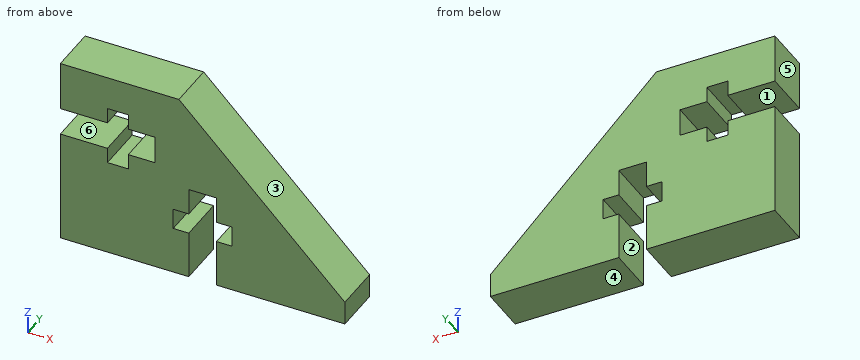
Autodesk Inventor part; units mm, degrees
ref_plane "Work Plane1" through (0, 0, 0) normal (0, 0, 1) x (1, 0, 0)
ref_plane "YZ Plane" through (0, 0, 0) normal (1, 0, 0) x (0, 1, 0)
ref_plane "XZ Plane" through (0, 0, 0) normal (0, 1, 0) x (-1, 0, 0)
ref_plane "Work Plane1" through (0, 0, 0) normal (0, 0, 1) x (1, 0, 0)
sketch "Sketch1" plane through (0, 0, 0) normal (0, 0, 1) x (1, 0, 0)
  line L0 (41.9864, 2.5) -> (43.4368, -2.0363) construction
  arc A0 (41.9864, 2.5) -> (43.4368, -2.0363) centre (41.9864, 0) ccw construction
  line L1 (112.0586, -28.575) -> (85.0037, -28.575) construction
  line L2 (112.0586, 28.1043) -> (112.0586, -28.575) construction
  line L3 (83.2959, 28.1043) -> (112.0586, 28.1043) construction
  arc A1 (83.2959, 28.1043) -> (1.0011, 28.575) centre (41.9864, 0) ccw construction
  line L4 (-116.5414, 28.575) -> (1.0011, 28.575) construction
  line L5 (-116.5414, -29.0493) -> (-116.5414, 28.575) construction
  line L6 (-0.7121, -29.0493) -> (-116.5414, -29.0493) construction
  arc A2 (-0.7121, -29.0493) -> (85.0037, -28.575) centre (41.9864, 0) ccw construction
  line L7 (-110.1914, 28.575) -> (-110.1914, 24.0792) construction
  line L8 (-111.9045, -9.9993) -> (-73.8045, -9.9993)
  line L9 (-73.8045, -9.9993) -> (-73.8045, -16.3493)
  line L10 (-73.8045, -16.3493) -> (-111.9045, -16.3493)
  line L11 (-111.9045, -16.3493) -> (-111.9045, -9.9993)
  circle A3 centre (88.3718, 12.2257) radius 1.8542
  circle A4 centre (108.8836, -22.6993) radius 1.8542
  circle A5 centre (-92.8545, -12.7) radius 1.8542
  circle A6 centre (-113.3664, 22.225) radius 1.8542
  circle A7 centre (-92.8545, 12.2257) radius 1.8542
  circle A8 centre (-113.3664, -22.6993) radius 1.8542
  circle A9 centre (88.3718, -12.7) radius 1.8542
  circle A10 centre (108.8836, 22.225) radius 1.8542
  point P0 (0, 0)
  dimension "d0" = 38.1
  dimension "d1" = 6.35
  dimension "d2" = 12.7
extrude "Extrusion1" add sketch "Sketch1" along normal blind 25.4 contours L8 L9 L10 L11 | A5
chamfer "Chamfer1" distance 22.225 angle 45 1 edges at (-73.8045, -13.1743, 25.4)
sketch "Sketch2" plane through (-111.9045, -16.3493, 0) normal (0, -1, 0) x (1, 0, 0)
  line L0 (38.1, 0) -> (0, 0)
  line L1 (17.1958, 0) -> (20.9042, 0)
  line L2 (19.05, 12.7239) -> (19.05, -0.6753) construction
  line L3 (17.1958, 12.7) -> (20.9042, 12.7)
  line L4 (20.9042, 12.7) -> (20.9042, 0)
  line L5 (20.9042, 0) -> (17.1958, 0)
  line L6 (17.1958, 0) -> (17.1958, 12.7)
  line L7 (15.113, 9.144) -> (22.987, 9.144)
  line L8 (22.987, 9.144) -> (22.987, 6.35)
  line L9 (22.987, 6.35) -> (15.113, 6.35)
  line L10 (15.113, 6.35) -> (15.113, 9.144)
  line L11 (0, 0) -> (0, 25.4)
  line L12 (12.7, 18.8338) -> (12.7, 15.1254)
  line L13 (12.7, 15.1254) -> (0, 15.1254)
  line L14 (0, 18.8338) -> (12.7, 18.8338)
  line L15 (9.0991, 20.9166) -> (9.0991, 13.0426)
  line L16 (9.0991, 13.0426) -> (6.3051, 13.0426)
  line L17 (6.3051, 13.0426) -> (6.3051, 20.9166)
  line L18 (6.3051, 20.9166) -> (9.0991, 20.9166)
  point P0 (111.9045, 0)
  dimension "d8" = 7.874
  dimension "d9" = 2.794
  dimension "d10" = 3.937
  dimension "d11" = 3.937
  dimension "d12" = 1.9733
  dimension "d13" = 1.9733
  dimension "d14" = 6.35
  dimension "d15" = 12.7
extrude "Extrusion2" cut sketch "Sketch2" against normal through all
equation "\"d10\" = d11"
equation "\"d13\" = d12"
properties part number "cornerBrace"
For this review, take the finished solid that the model builds, in its own axes (mm). Face numbers are marked on the shaded views. A direction names the side the tool comes from. Give positions to 0.01 mm unless a question says otherwise; leave off trailing zeros. Loops run counter-clockwise (first coordinate to the right, second up) from the corner with the lowest first, then second, coordinate; pieces in that order, holes last. Notation, with made-up numbers: M 15.5,-0.5 L 36.5,-0.5 A24 cw 36.5,18.5 Z; hole C 59.25,-29.75 d9. An arc over 180 degrees is marked long. Put each result on its own line as item: value. Start each with the question number.
(1) Machinability: for the marked faces 1, 2 and 3, which of the approach directions +Z, -Z, +X, -X, +Y, -Y give a long, thin tool a straight path to every point of the face, cutting with its end or side? Answer none if there is none.
(2) Add section D-D, the plane x = -93. Write out the cut boundary in (y, z), then the cut area to 3 significant figures.
(3) The part is to be moulded in two halves that separate along Z. For the marked faces 4, 5 and 6, say which applies: +Z half, -Z half, draft (parallel to the pull), parting line (faces both ways), or undercut.
(4) For pin 1 (2 mm diameter, centred on x = -104.5, y = -14, fed in from -Z); pin 2 (0.6 mm diameter, centred on y = -14.5, z = 19.5, fed in from +X); pin 3 (2 mm diameter, centred on y = -14.5, z = 8.5, fed in from +X); pin 4 (1.9 mm diameter, centred on x = -93, y = -13.5, fed in from -Z), all flat-tipped, find the tip position at first contact; note any pin that passes through.
(5) Add section A-A, the plane z = 2.5. Write out the cut boundary in (x, y).
(6) Add section B-B, the plane x = -101. Write out the cut boundary in (y, z).
(7) Wall thickness on L1, parallel to Z at x = -109.5, y = -15.5; L2, parallel to Z at x = -104, y = -11.25; L3, parallel to X at y = -14.5, z = 8.75: over which ranges is each line inside the solid? List them lowest first.
Result:
1. face 1: -X, +Y, -Y
1. face 2: -Z, +Y, -Y
1. face 3: +Z, +X, +Y, -Y
2. outline: M -16.35,12.7 L -10,12.7 L -10,22.37 L -16.35,22.37 Z
2. area: 61.4 mm^2
3. face 4: -Z half
3. face 5: draft
3. face 6: undercut
4. pin 1: stops at z = 0
4. pin 2: stops at x = -89.83
4. pin 3: stops at x = -78.13
4. pin 4: stops at z = 12.7
5. outline: M -111.9,-16.35 L -94.71,-16.35 L -94.71,-10 L -111.9,-10 Z; M -91,-16.35 L -73.8,-16.35 L -73.8,-10 L -91,-10 Z
6. outline: M -16.35,0 L -10,0 L -10,15.13 L -16.35,15.13 Z; M -16.35,18.83 L -10,18.83 L -10,25.4 L -16.35,25.4 Z
7. L1: z = 0 to 15.13, 18.83 to 25.4
7. L2: z = 0 to 13.04, 20.92 to 25.4
7. L3: x = -111.9 to -96.79, -88.92 to -79.38
